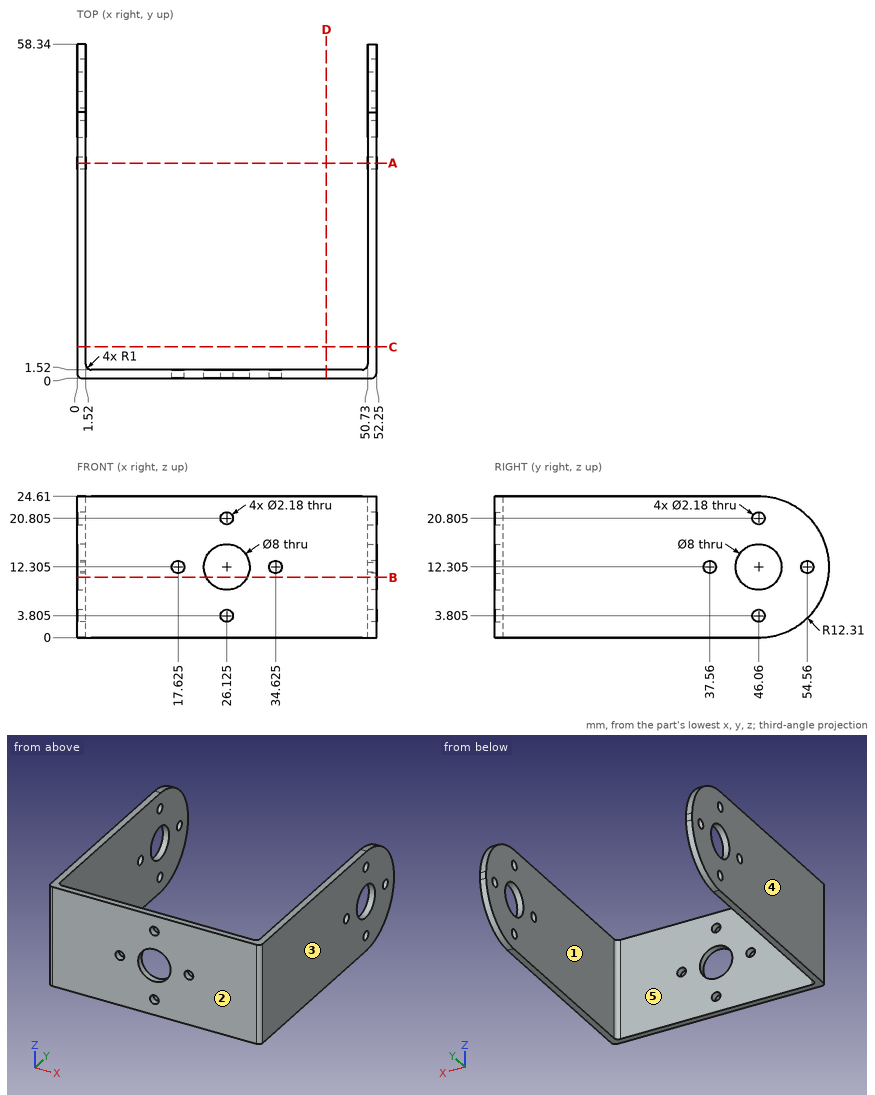
Check sheet for the drawn part. Datum: minimum x, y, z corner. Units: mm. A direction names the side the tool comes from. Round coordinates to 2 decimals unless told otherwise and drop trailing zeros. Loops run counter-clockwise (first coordinate to the right, second up) from the corner with the lowest first, then second, coordinate; pieces in that order, holes last.
Item 1: Cross-section at C-C on y = 5.5. Record the boundary of the cut face in (x, z), then the cut area to 3 significant figures.
Item 2: Mould release check, pull along X, two halves, no side actions. Record for the marked faces 3, 4 and 5: pulls with the +X half, pulls with the -X half, needs draft (parallel to the pull), parting line crosses it, or undercut.
Item 3: Cross-section at D-D on x = 43.5. Record the boundary of the cut face in (y, z), then the cut area to 3 significant figures.
Item 4: Cross-section at A-A on y = 37.56. Record the boundary of the cut face in (x, z) (3 decimals), then the cut area to 3 significant figures.
Item 5: Access from +Z, -Z, +X, -X, +Y, -Y to the whole of each face (thin tool, end or side, straight path). Record for the marked faces 1 and 2.
Item 6: Gauge pin test, flat ends, axial feed: pin 1 (12.5 mm diameter, centred on x = 19, z = 12, fed in from +Y); pin 2 (1.3 mm diameter, centred on y = 37.56, z = 12.305, fed in from -X); pin 3 (10 mm diameter, centred on x = 7, z = 10, fed in from +Y). Record the tip position at first contact, or that the pin passes through.
Item 7: Cross-section at B-B on z = 10.5. Record the boundary of the cut face in (x, y), then the cut area to 3 significant figures.
Item 8: Thickness scan on line 1 (X direction, y = 26, z = 18.25); line 2 (Y direction, x = 37, z = 4.25); line 3 (Y direction, x = 50, z = 16.25). Record the ranges inside material, lowest first.
Answer sheet:
1. outline: (0, 0) - (1.52, 0) - (1.52, 24.61) - (0, 24.61) - close; (50.73, 0) - (52.25, 0) - (52.25, 24.61) - (50.73, 24.61) - close
1. area: 74.8 mm2
2. face 3: pulls with the +X half
2. face 4: pulls with the -X half
2. face 5: undercut
3. outline: (0, 0) - (1.52, 0) - (1.52, 24.61) - (0, 24.61) - close
3. area: 37.4 mm2
4. outline: (0, 0) - (1.52, 0) - (1.52, 11.215) - (0, 11.215) - close; (0, 13.395) - (1.52, 13.395) - (1.52, 24.61) - (0, 24.61) - close; (50.73, 0) - (52.25, 0) - (52.25, 11.215) - (50.73, 11.215) - close; (50.73, 13.395) - (52.25, 13.395) - (52.25, 24.61) - (50.73, 24.61) - close
4. area: 68.2 mm2
5. face 1: +Z, -Z, +Y
5. face 2: +Z, -Z, +X, -X, -Y
6. pin 1: stops at y = 1.52
6. pin 2: passes through
6. pin 3: stops at y = 1.67
7. outline: (0, 1) arc R1 ccw to (1, 0) - (22.56, 0) - (22.56, 1.52) - (2.52, 1.52) arc R1 cw to (1.52, 2.52) - (1.52, 42.49) - (0, 42.49) - close; (0, 49.63) - (1.52, 49.63) - (1.52, 58.24) - (0, 58.24) - close; (29.69, 0) - (51.25, 0) arc R1 ccw to (52.25, 1) - (52.25, 42.49) - (50.73, 42.49) - (50.73, 2.52) arc R1 cw to (49.73, 1.52) - (29.69, 1.52) - close; (50.73, 49.63) - (52.25, 49.63) - (52.25, 58.24) - (50.73, 58.24) - close
7. area: 219 mm2
8. line 1: x = 0 to 1.52, 50.73 to 52.25
8. line 2: y = 0 to 1.52
8. line 3: y = 0 to 1.56
